from build123d import *

# Parameters (mm, degrees)
BOSS_EXTRUDE1_DEPTH                    = 6.35
SKETCH2_R                              = 10
CUT_EXTRUDE1_DEPTH                     = 153.884452556
M8_CLEARANCE_HOLE1_D                   = 9
M8_CLEARANCE_HOLE1_CSINK_D             = 9.05
M8_CLEARANCE_HOLE1_CSINK_ANGLE         = 90
CBORE_FOR_M5_HEX_HEAD_BOLT1_AT_2_COUNT = 2
CBORE_FOR_M5_HEX_HEAD_BOLT1_AT_2_PITCH = 19.798989873
CBORE_FOR_M5_HEX_HEAD_BOLT1_AT_3_COUNT = 2
CBORE_FOR_M5_HEX_HEAD_BOLT1_AT_3_PITCH = 36.769552622
CBORE_FOR_M5_HEX_HEAD_BOLT1_AT_4_COUNT = 2
CBORE_FOR_M5_HEX_HEAD_BOLT1_AT_4_PITCH = 20
CBORE_FOR_M5_HEX_HEAD_BOLT1_AT_5_COUNT = 2
CBORE_FOR_M5_HEX_HEAD_BOLT1_AT_5_PITCH = 36.769552622
CBORE_FOR_M5_HEX_HEAD_BOLT1_AT_6_COUNT = 2
CBORE_FOR_M5_HEX_HEAD_BOLT1_AT_6_PITCH = 48.083261121
FILLET1_R                              = 10


with BuildPart() as part:
    # Sketch1 → Boss-Extrude1 (new body)
    with BuildSketch(Plane(origin=(0, 0, 0), x_dir=(1, 0, 0), z_dir=(0, 1, 0))):
        Polygon((100, 57.735026919), (0, 115.470053838), (-100, 57.735026919), (-100, -57.735026919), (0, -115.470053838), (100, -57.735026919), align=None)
    extrude(amount=BOSS_EXTRUDE1_DEPTH)

    # Sketch2 → Cut-Extrude1 (cut, through all)
    with BuildSketch(Plane(origin=(0, 6.35, 0), x_dir=(1, 0, 0), z_dir=(0, 1, 0))):
        with Locations(Location((0, 0, 0), (0, 0, 270))):
            Circle(SKETCH2_R)
    extrude(amount=-CUT_EXTRUDE1_DEPTH, mode=Mode.SUBTRACT)

    # M8 Clearance Hole1 (through all)
    with Locations(Plane(origin=(0, 6.35, 0), x_dir=(1, 0, 0), z_dir=(0, 1, 0))):
        with Locations((0, 70), (0, 50), (0, -50), (0, -70)):
            CounterSinkHole(M8_CLEARANCE_HOLE1_D / 2, M8_CLEARANCE_HOLE1_CSINK_D / 2, counter_sink_angle=M8_CLEARANCE_HOLE1_CSINK_ANGLE)

    # Sketch8 → CBORE for M5 Hex Head Bolt1 (revolve, cut)
    with BuildSketch(Plane(origin=(-26, 6.35, -10), x_dir=(0, 0, 1), z_dir=(1, 0, 0))):
        Polygon((0, 0), (0, 6.35), (2.75, 6.35), (2.75, 3.58), (6.12, 3.58), (6.12, 0.025), (6.145, 0), align=None)
    cbore_for_m5_hex_head_bolt1 = revolve(axis=Axis((-26, 12.7, -10), (0, -1, 0)), mode=Mode.SUBTRACT)

    # CBORE for M5 Hex Head Bolt1 at 2: CBORE for M5 Hex Head Bolt1 ×2
    with Locations(*[Vector(0.7071067811865476, 0, -0.7071067811865476) * (i * CBORE_FOR_M5_HEX_HEAD_BOLT1_AT_2_PITCH) for i in range(1, CBORE_FOR_M5_HEX_HEAD_BOLT1_AT_2_COUNT)]):
        add(cbore_for_m5_hex_head_bolt1, mode=Mode.SUBTRACT)

    # CBORE for M5 Hex Head Bolt1 at 3: CBORE for M5 Hex Head Bolt1 ×2
    with Locations(*[Vector(0.924678098474716, 0, -0.38074980525429486) * (i * CBORE_FOR_M5_HEX_HEAD_BOLT1_AT_3_PITCH) for i in range(1, CBORE_FOR_M5_HEX_HEAD_BOLT1_AT_3_COUNT)]):
        add(cbore_for_m5_hex_head_bolt1, mode=Mode.SUBTRACT)

    # CBORE for M5 Hex Head Bolt1 at 4: CBORE for M5 Hex Head Bolt1 ×2
    with Locations(*[(0, 0, i * CBORE_FOR_M5_HEX_HEAD_BOLT1_AT_4_PITCH) for i in range(1, CBORE_FOR_M5_HEX_HEAD_BOLT1_AT_4_COUNT)]):
        add(cbore_for_m5_hex_head_bolt1, mode=Mode.SUBTRACT)

    # CBORE for M5 Hex Head Bolt1 at 5: CBORE for M5 Hex Head Bolt1 ×2
    with Locations(*[Vector(0.38074980525429486, 0, 0.924678098474716) * (i * CBORE_FOR_M5_HEX_HEAD_BOLT1_AT_5_PITCH) for i in range(1, CBORE_FOR_M5_HEX_HEAD_BOLT1_AT_5_COUNT)]):
        add(cbore_for_m5_hex_head_bolt1, mode=Mode.SUBTRACT)

    # CBORE for M5 Hex Head Bolt1 at 6: CBORE for M5 Hex Head Bolt1 ×2
    with Locations(*[Vector(0.7071067811865476, 0, 0.7071067811865476) * (i * CBORE_FOR_M5_HEX_HEAD_BOLT1_AT_6_PITCH) for i in range(1, CBORE_FOR_M5_HEX_HEAD_BOLT1_AT_6_COUNT)]):
        add(cbore_for_m5_hex_head_bolt1, mode=Mode.SUBTRACT)

    # Fillet1
    fillet1_edges = [part.edges().sort_by_distance(p)[0] for p in [
        (100, 3.175, 57.735026919),
        (0, 3.175, 115.470053838),
        (-100, 3.175, 57.735026919),
        (-100, 3.175, -57.735026919),
        (0, 3.175, -115.470053838),
        (100, 3.175, -57.735026919),
    ]]
    fillet(fillet1_edges, radius=FILLET1_R)


solid = part.part
Build history of the part. All positions in model axes, mm. A direction names the side the tool comes from. Coordinates: 2 decimals unless noted, no trailing zeros. Write each loop counter-clockwise with the first axis right and the second up, starting at its lowest first coordinate (ties: lowest second). Pieces come first, ordered by that corner, then holes. Notation, with made-up numbers: (-36, -22) -> (15, -22) arc R33 ccw to (15, 16) -> close; hole circle Ø8 at (75.25, -5). An arc over 180 degrees is marked (long way). Use CSV: the item, a comma, the result in double quotes. Start each with the question number.
Q1. Drill centre lines: probe 1 along X at (y, z) = (0.85, -24); probe 2 along X at (y, z) = (3.5, 8.5); probe 3 along Z at (x, y) = (12.5, 5.75). Where is each one in solid material? Low to high.
Q2. Cut at B-B, the plane z = -70. List the corners of the cut face in (x, y) (3 decimals).
Q3. 3-axis set-ups, long thin cutter, end or side, ignore diameter. For faces 4 (the flat face through (11, 2.77, 23)), 5 (the cylindrical face through (0.59, 3.12, -74.46)): which of +Z, -Z, +X, -X, +Y, -Y reach the whole face in a straight line?
Q4. Cut at D-D, the plane z = 89. List the corners of the cut face in (x, y).
Q5. Flat gauge pins, fed straight in: pin 1 Ø4.5 at (x, z) = (-12, -24) entering from -Y; pin 2 Ø14.5 at (x, z) = (0, -70) entering from +Y; pin 3 Ø1.5 at (y, z) = (4, -73.5) entering from -X; pin 4 Ø6 at (x, z) = (9, -25) entering from +Y. Where does each tip first touch, or does it go through?
Q6. Pull direction Z, two halves, no side cores. Call faces 1 (the cylindrical face through (-22.28, 4.57, -14.86)), 2 (the flat face through (100, 3, 1)), 3 (the flat face through (49.37, 3.131, 86.966)): released by +Z, released by -Z, zero draft, split by the parting line, or undercut.
Q7. Cut at C-C, the plane x = -45. List the corners of the cut face in (y, z).
Q8. Cut at A-A, the plane y = 1.25. State how many separate pieces and enclosed holes the cut face has, then the cut area to 3 significant figures.
Checked values:
1,probe 1,"x = -100 to -14.75, -9.25 to 5.25, 10.75 to 100"
1,probe 2,"x = -100 to -31.93, -20.07 to -5.27, 5.27 to 100"
1,probe 3,"z = -108.25 to -28.15, -19.85 to 19.85, 28.15 to 108.25"
2,outline,"(-78.756, 0) -> (-4.5, 0) -> (-4.5, 6.325) -> (-4.525, 6.35) -> (-78.756, 6.35) -> close; (4.5, 0) -> (78.756, 0) -> (78.756, 6.35) -> (4.525, 6.35) -> (4.5, 6.325) -> close"
3,face 4,"+Y"
3,face 5,"+Y, -Y"
4,outline,"(-45.85, 0) -> (45.85, 0) -> (45.85, 6.35) -> (-45.85, 6.35) -> close"
5,pin 1,"passes through"
5,pin 2,"stops at y = 6.35"
5,pin 3,"stops at x = -73.99"
5,pin 4,"stops at y = 2.77"
6,face 1,"undercut"
6,face 2,"zero draft"
6,face 3,"released by +Z"
7,outline,"(0, -89.49) -> (6.35, -89.49) -> (6.35, 89.49) -> (0, 89.49) -> close"
8,separate pieces,"1"
8,enclosed holes,"11"
8,area,"33,900 mm²"
